```python
from build123d import *

# Parameters (mm, degrees)
F1_DEPTH = 63.5
F0_W     = 25.4
F0_H     = 19.05
F2_DEPTH = 25.4
F3_DEPTH = 7.9375
F4_R     = 5.08
F6_R     = 6.35
F7_DEPTH = 50.8
F8_R     = 19.05
F9_DEPTH = 25.4


with BuildPart() as f1:
    # F0 (on Front) → F1 (new body, symmetric)
    with BuildSketch(Plane.XZ):
        Polygon((-41.275, -9.525), (41.275, -9.525), (41.275, 9.525), (22.225, 9.525), (-41.275, 9.525), align=None)
    extrude(amount=F1_DEPTH, both=True)

    # F0 (on Front) → F2 (join, symmetric)
    with BuildSketch(Plane.XZ):
        with BuildLine():
            Line((22.225, 9.525), (41.275, 9.525))
            Line((41.275, 9.525), (41.275, 27.0002))
            ThreePointArc((41.275, 27.0002), (45.9246798487, 38.2255201513), (57.15, 42.8752))
            Line((57.15, 42.8752), (60.325, 42.8752))
            Line((60.325, 42.8752), (60.325, 61.9252))
            Line((60.325, 61.9252), (57.15, 61.9252))
            add(Edge.make_bspline(
                [(54.3558038177, 61.8132448639), (55.2992353906, 61.8602813509), (56.2310037171, 61.8975367589), (57.15, 61.9252)],
                knots=[108.500811641, 108.500811641, 108.500811641, 108.500811641, 111.5045361635, 111.5045361635, 111.5045361635, 111.5045361635], degree=3))
            ThreePointArc((54.3558038177, 61.8132448639), (31.4854044775, 50.6874151522), (22.225, 27.0002))
            Line((22.225, 27.0002), (22.225, 9.525))
        make_face()
        with Locations((73.025, 52.4002)):
            Rectangle(F0_W, F0_H)
    extrude(amount=F2_DEPTH, both=True)

    # F0 (on Front) → F3 (join, symmetric)
    with BuildSketch(Plane.XZ):
        with BuildLine():
            add(Edge.make_bspline(
                [(-41.275, 9.525), (-29.0199070695, 45.652726812), (20.2770823423, 60.114188583), (54.3558038177, 61.8132448639)],
                knots=[0, 0, 0, 0, 108.500811641, 108.500811641, 108.500811641, 108.500811641], degree=3))
            Line((-41.275, 9.525), (22.225, 9.525))
            Line((22.225, 9.525), (22.225, 27.0002))
            ThreePointArc((22.225, 27.0002), (31.4854044775, 50.6874151522), (54.3558038177, 61.8132448639))
        make_face()
    extrude(amount=F3_DEPTH, both=True)

    # F4
    f4_edges = [f1.edges().sort_by_distance(p)[0] for p in [
        (41.275, -63.5, 0),
        (-41.275, -63.5, 0),
        (-41.275, 63.5, 0),
        (41.275, 63.5, 0),
    ]]
    fillet(f4_edges, radius=F4_R)

    # F0 (on Front) → F5 (revolve)
    with BuildSketch(Plane.XZ):
        Polygon((85.725, 61.9252), (85.725, 42.8752), (85.725, 38.1), (111.125, 38.1), (111.125, 66.675), (85.725, 66.675), align=None)
    revolve(axis=Axis((85.725, 0, 52.3875), (0, 0, -1)))

    # F6 (on face) → F7 (cut, symmetric)
    with BuildSketch(Plane.XY.offset(9.525)):
        with Locations((29.4948853552, 51.6811832786)):
            Circle(F6_R)
    extrude(amount=F7_DEPTH, both=True, mode=Mode.SUBTRACT)

    # F8 (on face) → F9 (cut)
    with BuildSketch(Plane.XY.offset(66.675)):
        with Locations((85.725, 0)):
            Circle(F8_R)
    extrude(amount=-F9_DEPTH, mode=Mode.SUBTRACT)


solid = f1.part
```
Geometry: final body of the model. Coordinates: model frame, mm. A direction names the side the tool comes from. Give positions to 0.01 mm unless a question says otherwise; leave off trailing zeros. Loops run counter-clockwise (first coordinate to the right, second up) from the corner with the lowest first, then second, coordinate; pieces in that order, holes last. Notation, with made-up numbers: (11.25, -40) -> (40.25, -40) arc R5 ccw to (40.25, -33) -> close; hole circle Ø10 at (87.5, 30). An arc over 180 degrees is marked (long way). Use one line per item in the form item = value.
Item 1: Access query for faces 1 (the face through (46, -25.4, 42)), 2 (the face through (31.73, 16.55, 50.95)), 3 (the face through (-3, -7.938, 30)), 4 (the face through (103.895, 5.722, 54.153)). Directions: +Z, -Z, +X, -X, +Y, -Y. A direction counts if a zero-diameter tool reaches every point of the face in a straight line with its end or side. Return the directions, or none.
A:
face_1 = +Z, +X, -X, -Y
face_2 = +Z, -X, +Y
face_3 = +Z, -X, -Y
face_4 = +Z
Item 2: Section query A-A on y = 49. Output: boundary loops of the cut face in (x, z) (3 decimals).
A:
outline = (-41.275, -9.525) -> (23.739, -9.525) -> (23.739, 9.525) -> (-41.275, 9.525) -> close; (35.251, -9.525) -> (41.275, -9.525) -> (41.275, 9.525) -> (35.251, 9.525) -> close
Item 3: Section query D-D on y = -46. Output: boundary loops of the cut face in (x, z) (3 decimals), and give its area (3 significant figures).
A:
outline = (-41.275, -9.525) -> (41.275, -9.525) -> (41.275, 9.525) -> (-41.275, 9.525) -> close
area = 1,570 mm^2
Item 4: Line query: probe 1 along X at (y, z) = (-18.5, -2) (3 decimals); probe 2 along Z at (x, y) = (2, 37) (3 decimals); probe 3 along Z at (x, y) = (81.5, -14) (3 decimals). Output: solid intervals per line, ascending.
A:
probe_1 = -41.275 to 41.275
probe_2 = -9.525 to 9.525
probe_3 = 38.1 to 41.275
Item 5: Draft query along X for faces 5 (the face through (41.275, -1, 4)), 6 (the face through (-1, 63.5, 0)), 7 (the face through (60, 2, 42.875)), 8 (the face through (31.73, -16.79, 50.95)). Return one class per face: pulls with the +X half, pulls with the -X half, needs draft (parallel to the pull), parting line crosses it, or undercut.
A:
face_5 = pulls with the +X half
face_6 = needs draft
face_7 = undercut
face_8 = pulls with the -X half
Item 6: Section query C-C on x = 82. Output: boundary loops of the cut face in (y, z) (3 decimals).
A:
outline = (-25.4, 42.875) -> (-25.125, 42.875) -> (-25.125, 38.1) -> (25.125, 38.1) -> (25.125, 42.875) -> (25.4, 42.875) -> (25.4, 61.925) -> (25.125, 61.925) -> (25.125, 66.675) -> (18.682, 66.675) -> (18.682, 41.275) -> (-18.682, 41.275) -> (-18.682, 66.675) -> (-25.125, 66.675) -> (-25.125, 61.925) -> (-25.4, 61.925) -> close
Item 7: Pin query (flat end, axial travel): P1, Ø15.5, axis at x = -10.5, z = 23, coming from the -Y side; P2, Ø1.5, axis at x = 18.5, z = 24, coming from the +Y side; P3, Ø23, axis at x = 69.5, y = 12, coming from the -Z side. Return the tip coordinate at first contact, or that it passes through.
A:
P1 = -7.94
P2 = 7.94
P3 = 38.1
Item 8: Section query B-B on z = 0.5. Output: boundary loops of the cut face in (x, y) (3 decimals), and give its area (3 significant figures).
A:
outline = (-41.275, -58.42) arc R5.08 ccw to (-36.195, -63.5) -> (36.195, -63.5) arc R5.08 ccw to (41.275, -58.42) -> (41.275, 58.42) arc R5.08 ccw to (36.195, 63.5) -> (-36.195, 63.5) arc R5.08 ccw to (-41.275, 58.42) -> close; hole circle Ø12.7 at (29.495, 51.681)
area = 10,300 mm^2
